Model file for the job. Use its own axes, mm. Face numbers are marked on the shaded views. A direction names the side the tool comes from. Coordinates: 2 decimals unless noted, no trailing zeros. Order: outer loops, then holes, each group sorted by start corner. A loop starts at its lowest first (then second) coordinate and runs counter-clockwise, first axis right, second up. Notation, with made-up numbers: (-39, -4) -> (12, -4) arc R17 ccw to (12, 23) -> close; hole circle Ø2 at (67, 22). An arc over 180 degrees is marked (long way). Write item = value, one per line. Start each with the question number.
Q1. Cut at A-A, the plane y = 12.7. List the corners of the cut face in (x, z) (3 decimals), plus the area to 3 significant figures.
Q2. Mould opens along Y. For the marked faces 1, 2 and 3 say: +Y half, -Y half, draft (parallel to the pull), parting line (faces both ways), or undercut.
Q3. Cut at C-C, the plane x = 0. List the corners of the cut face in (y, z) (3 decimals), plus the area to 3 significant figures.
Q4. Flat gauge pins, fed straight in: pin 1 (3 mm diameter, centred on x = -5, z = -8, fed in from -Y); pin 2 (10 mm diameter, centred on x = 3.5, y = 24, fed in from -Z); pin 3 (5 mm diameter, centred on y = 12.7, z = 0, fed in from +X). Where does each tip first touch, or does it go through?
Q5. Cut at D-D, the plane y = 6.5. List the corners of the cut face in (x, z) (3 decimals).
Q6. Cut at B-B, the plane z = 0. List the corners of the cut face in (x, y) (3 decimals), plus the area to 3 significant figures.
Q7. 3-axis set-ups, long thin cutter, end or side, ignore diameter. For the marked faces 4 and 5: which of +Z, -Z, +X, -X, +Y, -Y reach the whole face in a straight line?
Q8. Wall check: line 1 (X direction, y = 12.5, z = 11.5) (3 decimals); line 2 (Z direction, x = 0, y = 27.6) (3 decimals); line 3 (Y direction, x = 2.5, z = -11). Give the ranges that are in metal, low to high. Write a range as from..to.
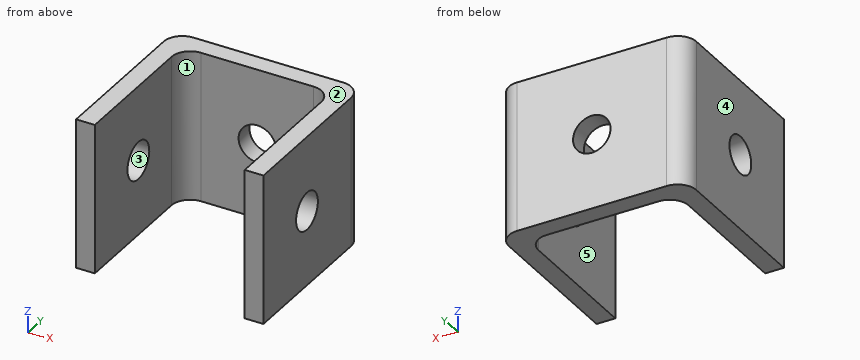
Autodesk Inventor part; units mm, degrees
ref_plane "YZ Plane" through (0, 0, 0) normal (1, 0, 0) x (0, 1, 0)
ref_plane "XZ Plane" through (0, 0, 0) normal (0, 1, 0) x (-1, 0, 0)
ref_plane "XY Plane" through (0, 0, 0) normal (0, 0, 1) x (1, 0, 0)
sketch "Sketch1" plane through (0, 0, 0) normal (0, 0, 1) x (1, 0, 0)
  line L0 (-15.875, 0) -> (-12.7, 0)
  line L1 (-12.7, 0) -> (-12.7, 22.352)
  line L2 (-9.525, 25.527) -> (9.525, 25.527)
  line L3 (12.7, 22.352) -> (12.7, 0)
  line L4 (12.7, 0) -> (15.875, 0)
  line L5 (15.875, 0) -> (15.875, 25.527)
  line L6 (12.7, 28.702) -> (-12.7, 28.702)
  line L7 (-15.875, 25.527) -> (-15.875, 0)
  arc A0 (-9.525, 25.527) -> (-12.7, 22.352) centre (-9.525, 22.352) ccw
  arc A1 (12.7, 22.352) -> (9.525, 25.527) centre (9.525, 22.352) ccw
  arc A2 (-12.7, 28.702) -> (-15.875, 25.527) centre (-12.7, 25.527) ccw
  arc A3 (15.875, 25.527) -> (12.7, 28.702) centre (12.7, 25.527) ccw
  line L8 (0, 35.2315) -> (0, -5.8719)
  point P0 (0, 0)
  dimension "d0" = 28.702
  dimension "d1" = 31.75
  dimension "d2" = 3.175
  dimension "d3" = 3.175
  dimension "d4" = 3.175
extrude "Extrusion1" add sketch "Sketch1" along normal mid plane 25.4
sketch "Sketch4" plane through (15.875, 0, 12.7) normal (1, 0, 0) x (0, 0, -1)
  line L0 (12.7, -5.7404) -> (12.7, 34.4424) construction
  line L1 (-140.335, 0) -> (842.01, 0) construction
  circle A0 centre (12.7, 12.7) radius 3.175
  point P0 (12.7, 0)
  dimension "d34" = 12.7
  dimension "d35" = 0
  dimension "d36" = 6.35
extrude "Extrusion4" cut sketch "Sketch4" against normal up to surface (31.75 mm away)
pattern_linear "Rectangular Pattern3" count 30 spacing 25.4 along (0, 0, 1) count 30 spacing 25.4 along (0, 0, -1) of "Extrusion4"
sketch "Sketch5" plane through (-12.7, 28.702, 12.7) normal (0, 1, 0) x (1, 0, 0)
  circle A0 centre (12.7, 12.7) radius 3.175
  dimension "d45" = 6.35
extrude "Extrusion5" cut sketch "Sketch5" against normal up to next
equation "\"d5\" = AdaptLength"
equation "\"AdaptLength\" = 25.4"
properties part number "NSupportChannel2"
Here are the results:
q1.outline = (-15.875, -12.7) -> (-12.7, -12.7) -> (-12.7, -3.175) -> (-15.875, -3.175) -> close; (-15.875, 3.175) -> (-12.7, 3.175) -> (-12.7, 12.7) -> (-15.875, 12.7) -> close; (12.7, -12.7) -> (15.875, -12.7) -> (15.875, -3.175) -> (12.7, -3.175) -> close; (12.7, 3.175) -> (15.875, 3.175) -> (15.875, 12.7) -> (12.7, 12.7) -> close
q1.area = 121 mm²
q2.face_1 = -Y half
q2.face_2 = draft
q2.face_3 = undercut
q3.outline = (25.527, -12.7) -> (28.702, -12.7) -> (28.702, -3.175) -> (25.527, -3.175) -> close; (25.527, 3.175) -> (28.702, 3.175) -> (28.702, 12.7) -> (25.527, 12.7) -> close
q3.area = 60.5 mm²
q4.pin_1 = 25.53
q4.pin_2 = -12.7
q4.pin_3 = through
q5.outline = (-15.875, -12.7) -> (-12.7, -12.7) -> (-12.7, 12.7) -> (-15.875, 12.7) -> close; (12.7, -12.7) -> (15.875, -12.7) -> (15.875, 12.7) -> (12.7, 12.7) -> close
q6.outline = (-15.875, 0) -> (-12.7, 0) -> (-12.7, 9.525) -> (-15.875, 9.525) -> close; (-15.875, 15.875) -> (-12.7, 15.875) -> (-12.7, 22.352) arc R3.175 cw to (-9.525, 25.527) -> (-3.175, 25.527) -> (-3.175, 28.702) -> (-12.7, 28.702) arc R3.175 ccw to (-15.875, 25.527) -> close; (3.175, 25.527) -> (9.525, 25.527) arc R3.175 cw to (12.7, 22.352) -> (12.7, 15.875) -> (15.875, 15.875) -> (15.875, 25.527) arc R3.175 ccw to (12.7, 28.702) -> (3.175, 28.702) -> close; (12.7, 0) -> (15.875, 0) -> (15.875, 9.525) -> (12.7, 9.525) -> close
q6.area = 202 mm²
q7.face_4 = +Z, -Z, -X, +Y, -Y
q7.face_5 = +Z, -Z, -Y
q8.line_1 = -15.875..-12.7, 12.7..15.875
q8.line_2 = -12.7..-3.175, 3.175..12.7
q8.line_3 = 25.53..28.7
